Geometry check sheet. Reference: the model listing, model coordinates, mm. A direction names the side the tool comes from. Round coordinates to 2 decimals unless told otherwise and drop trailing zeros. Order: outer loops, then holes, each group sorted by start corner. A loop starts at its lowest first (then second) coordinate and runs counter-clockwise, first axis right, second up.
(1) Go/stop test with flat-tipped pins: pin 1 (1 mm diameter, centred on y = 1.5, z = 2, fed in from +X); pin 2 (1.5 mm diameter, centred on x = -16, z = 2, fed in from +Y); pin 3 (12 mm diameter, centred on y = -2, z = -4, fed in from -X). Record where each tip stops, or that it passes through.
(2) Sectioned sample at A-A (y = 4). Record the boundary of the cut face in (x, z).
(3) Material ranges on line 1 along Y through (x, z) = (6, 1.5); line 2 along Y through (x, z) = (3, -1.25); line 3 along X through (y, z) = (2, -4.25), recorded low to high.
(4) Sectioned sample at B-B (z = -2.5). Record the boundary of the cut face in (x, y), plus the area to 3 significant figures.
(5) Sectioned sample at D-D (z = -8). Record the boundary of the cut face in (x, y), plus the area to 3 significant figures.
(6) Sectioned sample at C-C (x = -11.5). Record the boundary of the cut face in (y, z).
(7) Set-up check for faces 1 (the face through (0.87, 6.81, 4.93)), 2 (the face through (-6.45, -15.22, 4.93)), 3 (the face through (0.87, 6.81, -4.93)): record each of +Z, -Z, +X, -X, +Y, -Y from which the full face is reachable in a straight line by a thin tool's end or side.
from build123d import *

# Parameters (mm, degrees)
EXTRUDE_1_DEPTH       = 10
EXTRUDE_1_DRAFT       = 10
MIRROR_1_COPY_1_DEPTH = 10
MIRROR_1_COPY_1_DRAFT = 10
SKETCH_4_W            = 44.504913076
SKETCH_4_H            = 42.19047619
CUT_EXTRUDE_4_DEPTH   = 50


with BuildPart() as part:
    # 草图2 → 凸台-拉伸1 (with draft: the straight prism first)
    with BuildSketch(Plane.XY):
        Polygon((0, 0), (-30, -40), (10, 0), (10, 20), (0, 20), align=None)
    extrude(amount=EXTRUDE_1_DEPTH)
    # 凸台-拉伸1: the draft: its side faces are tilted about the plane it starts from
    extrude_1_sides = [part.faces().sort_by_distance(p)[0] for p in [
        (-15, -20, 5),
        (-10, -20, 5),
        (10, 10, 5),
        (5, 20, 5),
        (0, 10, 5),
    ]]
    draft(extrude_1_sides, Plane.XY, EXTRUDE_1_DRAFT)


with BuildPart() as mirror_1_copy_1_tool:
    # 镜向1 copy 1 sketch → 镜向1 copy 1 (with draft: the straight prism first)
    with BuildSketch(Plane(origin=(0, 0, 0), x_dir=(1, 0, 0), z_dir=(0, 0, -1))):
        Polygon((0, 0), (-30, 40), (10, 0), (10, -20), (0, -20), align=None)
    extrude(amount=MIRROR_1_COPY_1_DEPTH)
    # 镜向1 copy 1: the draft: its side faces are tilted about the plane it starts from
    mirror_1_copy_1_sides = [mirror_1_copy_1_tool.faces().sort_by_distance(p)[0] for p in [
        (-15, -20, -5),
        (-10, -20, -5),
        (10, 10, -5),
        (5, 20, -5),
        (0, 10, -5),
    ]]
    draft(mirror_1_copy_1_sides, Plane(origin=(0, 0, 0), x_dir=(1, 0, 0), z_dir=(0, 0, -1)), MIRROR_1_COPY_1_DRAFT)


with BuildPart() as part_1:
    add(part.part)

    # 镜向1 copy 1: add mirror_1_copy_1_tool
    add(mirror_1_copy_1_tool.part)

    # 草图4 → 切除-拉伸4 (cut, symmetric)
    with BuildSketch(Plane.XY):
        with Locations((4.175676145, 35.095238095)):
            Rectangle(SKETCH_4_W, SKETCH_4_H)
    extrude(amount=CUT_EXTRUDE_4_DEPTH, both=True, mode=Mode.SUBTRACT)


solid = part_1.part
Answer below:
1. pin 1: stops at x = 9.74
1. pin 2: stops at y = -20.9
1. pin 3: stops at x = -5.31
2. outline: (0, 0) - (1.76, -10) - (8.24, -10) - (10, 0) - (8.24, 10) - (1.76, 10) - close
3. line 1: y = -3.63 to 14
3. line 2: y = -6.69 to 14
3. line 3: x = 0.75 to 9.25
4. outline: (-25.93, -35.3) - (9.56, 0.18) - (9.56, 14) - (0.44, 14) - (0.44, -0.15) - close
4. area: 283 mm2
5. outline: (-16.96, -24.97) - (8.59, 0.58) - (8.59, 14) - (1.41, 14) - (1.41, -0.47) - close
5. area: 178 mm2
6. outline: (-21.5, 0) - (-19.01, -10) - (-18.27, -10) - (-15.33, 0) - (-18.27, 10) - (-19.01, 10) - close
7. face 1: +Z, -X, +Y
7. face 2: +Z, +X, -Y
7. face 3: -Z, -X, +Y
